Autodesk Inventor part; units mm, degrees
ref_plane "YZ Plane" through (0, 0, 0) normal (1, 0, 0) x (0, 1, 0)
ref_plane "XZ Plane" through (0, 0, 0) normal (0, 1, 0) x (-1, 0, 0)
ref_plane "XY Plane" through (0, 0, 0) normal (0, 0, 1) x (1, 0, 0)
sketch "Sketch1" plane through (0, 0, 0) normal (0, 1, 0) x (-1, 0, 0)
  line L0 (8.5, 11) -> (-8.5, 11)
  line L1 (-8.5, 11) -> (-8.5, -11)
  line L2 (-8.5, -11) -> (8.5, -11)
  line L3 (8.5, -11) -> (8.5, 11)
  line L4 (8.5, 11) -> (-8.5, -11) construction
  line L5 (-8.5, 11) -> (8.5, -11) construction
  point P0 (0, 0)
  dimension "d0" = 17
  dimension "d1" = 22
extrude "Body" add sketch "Sketch1" along normal blind 2
sketch "Sketch3" plane through (0, 2, 0) normal (0, 1, 0) x (1, 0, 0)
  line L0 (8.5, 11) -> (-8.5, 11)
  line L1 (0, 11) -> (0, -11)
  line L2 (-8.5, -11) -> (8.5, -11)
  line L3 (-2, -10) -> (-0.5, -10)
  line L4 (-0.5, -10) -> (-0.5, 10)
  line L5 (-0.5, 10) -> (-2, 10)
  line L6 (-2, 10) -> (-2, -10)
  line L7 (-2, -10) -> (-0.5, 10) construction
  line L8 (-0.5, -10) -> (-2, 10) construction
  line L9 (-4.25, 10) -> (-2.75, 10)
  line L10 (-2.75, 10) -> (-2.75, -10)
  line L11 (-2.75, -10) -> (-4.25, -10)
  line L12 (-4.25, -10) -> (-4.25, 10)
  line L13 (-4.25, 10) -> (-2.75, -10) construction
  line L14 (-2.75, 10) -> (-4.25, -10) construction
  line L15 (-8.5, 11) -> (-8.5, -11)
  line L16 (-8.5, 0) -> (8.5, 0)
  line L17 (-6.55, 10) -> (-5.05, 10)
  line L18 (-5.05, 10) -> (-5.05, -10)
  line L19 (-5.05, -10) -> (-6.55, -10)
  line L20 (-6.55, -10) -> (-6.55, 10)
  line L21 (-6.55, 10) -> (-5.05, -10) construction
  line L22 (-5.05, 10) -> (-6.55, -10) construction
  line L23 (2, -10) -> (0.5, -10)
  line L24 (0.5, -10) -> (0.5, 10)
  line L25 (0.5, 10) -> (2, 10)
  line L26 (2, 10) -> (2, -10)
  line L27 (2, -10) -> (0.5, 10) construction
  line L28 (0.5, -10) -> (2, 10) construction
  line L29 (4.25, 10) -> (2.75, 10)
  line L30 (2.75, 10) -> (2.75, -10)
  line L31 (2.75, -10) -> (4.25, -10)
  line L32 (4.25, -10) -> (4.25, 10)
  line L33 (4.25, 10) -> (2.75, -10) construction
  line L34 (2.75, 10) -> (4.25, -10) construction
  line L35 (6.55, 10) -> (5.05, 10)
  line L36 (5.05, 10) -> (5.05, -10)
  line L37 (5.05, -10) -> (6.55, -10)
  line L38 (6.55, -10) -> (6.55, 10)
  line L39 (6.55, 10) -> (5.05, -10) construction
  line L40 (5.05, 10) -> (6.55, -10) construction
  point P0 (0, 0)
  point P1 (-1.25, 0)
  point P2 (-3.5, 0)
  point P3 (-5.8, 0)
  point P4 (1.25, 0)
  point P5 (3.5, 0)
  point P6 (5.8, 0)
  dimension "d6" = 1.5
  dimension "d7" = 20
  dimension "d9" = 0.5
  dimension "d11" = 2.75
  dimension "d12" = 5.05
extrude "Rungs" cut sketch "Sketch3" against normal through all contours L36 L35 L38 L16 | L16 L38 L37 L36 | L30 L29 L32 L16 | L16 L32 L31 L30 | L24 L25 L26 L16 | L16 L26 L23 L24 | L16 L6 L5 L4 | L4 L3 L6 L16 | L20 L17 L18 L16 | L16 L18 L19 L20 | L16 L12 L9 L10 | L10 L11 L12 L16
sketch "Sketch4" plane through (0, 2, 0) normal (0, 1, 0) x (1, 0, 0)
  line L0 (0.5, -10) -> (0.5, 10)
  line L1 (-2, 10) -> (-0.5, 10)
  line L2 (0.5, -10) -> (-0.5, -10)
  line L3 (-0.5, -10) -> (-0.5, 10)
  line L4 (-0.5, 10) -> (0.5, 10)
  line L5 (0.5, 10) -> (0.5, -10)
  point P0 (0, 0)
extrude "Remove center rung" cut sketch "Sketch4" against normal through all
properties part number "jtd_tack_no_middle_20170113"
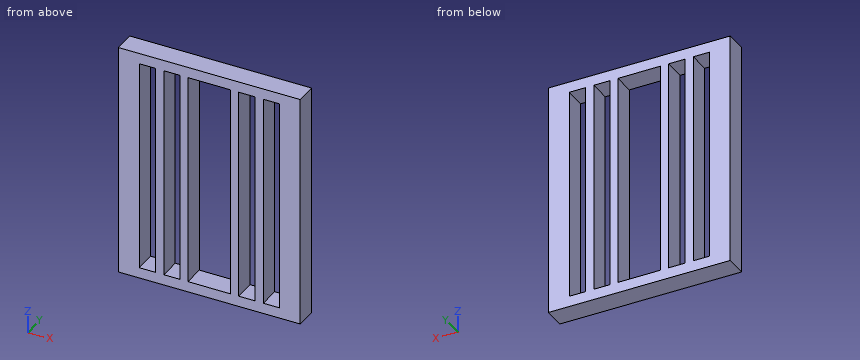
Can you work these out from the model? Positions are in its coordinate system, mm. Coordinates: 2 decimals unless noted, no trailing zeros. Order: outer loops, then holes, each group sorted by start corner. A loop starts at its lowest first (then second) coordinate and runs counter-clockwise, first axis right, second up. Notation, with made-up numbers: M 67,74.5 L 89,74.5 A16 cw 89,105.5 Z; hole C 81.5,26.5 d7. An arc over 180 degrees is marked long. Answer as CSV lines item,"result".
(1) Suppose I cut it at C-C on y = 0.95. Please give me the cut outline in (x, z), plus the area to 3 significant figures.
Geometry check:
outline,"M -8.5,-11 L 8.5,-11 L 8.5,11 L -8.5,11 Z; hole M -6.55,-10 L -5.05,-10 L -5.05,10 L -6.55,10 Z; hole M -4.25,-10 L -2.75,-10 L -2.75,10 L -4.25,10 Z; hole M -2,-10 L 2,-10 L 2,10 L -2,10 Z; hole M 2.75,-10 L 4.25,-10 L 4.25,10 L 2.75,10 Z; hole M 5.05,-10 L 6.55,-10 L 6.55,10 L 5.05,10 Z"
area,"174 mm^2"
(2) Suppose I cut it at B-B on z = -1. Please give me the cut outline in (x, y).
Geometry check:
outline,"M -8.5,0 L -6.55,0 L -6.55,2 L -8.5,2 Z; M -5.05,0 L -4.25,0 L -4.25,2 L -5.05,2 Z; M -2.75,0 L -2,0 L -2,2 L -2.75,2 Z; M 2,0 L 2.75,0 L 2.75,2 L 2,2 Z; M 4.25,0 L 5.05,0 L 5.05,2 L 4.25,2 Z; M 6.55,0 L 8.5,0 L 8.5,2 L 6.55,2 Z"
(3) Please list where these lines run through material, in increasing order: L1, parallel to X at y = 1.45, z = -5.25; L2, parallel to Z at x = 0.75, y = 0.4.
Geometry check:
L1,"-8.5 to -6.55, -5.05 to -4.25, -2.75 to -2, 2 to 2.75, 4.25 to 5.05, 6.55 to 8.5"
L2,"-11 to -10, 10 to 11"
(4) Suppose I cut it at A-A on x = 1.25. Please give me the cut outline in (y, z), plus the area to 3 significant figures.
Geometry check:
outline,"M 0,-11 L 2,-11 L 2,-10 L 0,-10 Z; M 0,10 L 2,10 L 2,11 L 0,11 Z"
area,"4.00 mm^2"
